For this review, take the finished solid that the model builds, in its own axes (mm). A direction names the side the tool comes from. Coordinates: 2 decimals unless noted, no trailing zeros. Loops run counter-clockwise (first coordinate to the right, second up) from the corner with the lowest first, then second, coordinate; pieces in that order, holes last. Notation, with made-up numbers: (12.25, 56.5) -> (45.25, 56.5) arc R27 ccw to (45.25, 74.5) -> close; hole circle Ø3 at (64, 45). An arc over 180 degrees is marked (long way). One line per item, written item: value.
from build123d import *

# Parameters (mm, degrees)
SKETCH_1_R               = 16.5
EXTRUDE_1_DEPTH          = 2.5
SKETCH_2_R               = 9.5
EXTRUDE_2_DEPTH          = 1.4
SKETCH_3_R               = 1.5
CUT_EXTRUDE_1_DEPTH      = 3
SKETCH_4_R               = 8.5
EXTRUDE_3_DEPTH          = 10
PATTERN_CIRCULAR_1_COUNT = 4
SKETCH_8_R               = 3
EXTRUDE_4_DEPTH          = 6
SKETCH_9_R               = 3.25
CUT_EXTRUDE_2_DEPTH      = 0.5


with BuildPart() as part:
    # 草图1 → 凸台-拉伸1 (new body)
    with BuildSketch(Plane.XY):
        Circle(SKETCH_1_R)
    extrude(amount=EXTRUDE_1_DEPTH)

    # 草图2 → 凸台-拉伸2 (add)
    with BuildSketch(Plane.XY.offset(2.5)):
        Circle(SKETCH_2_R)
    extrude(amount=EXTRUDE_2_DEPTH)

    # 草图3 → 切除-拉伸1 (cut)
    with BuildSketch(Plane.XY.offset(2.5)):
        with Locations((0, 13.5)):
            Circle(SKETCH_3_R)
        with Locations((11.691342951, 6.75)):
            Circle(SKETCH_3_R)
        with Locations((11.691342951, -6.75)):
            Circle(SKETCH_3_R)
        with Locations((0, -13.5)):
            Circle(SKETCH_3_R)
        with Locations((-11.691342951, -6.75)):
            Circle(SKETCH_3_R)
        with Locations((-11.691342951, 6.75)):
            Circle(SKETCH_3_R)
    extrude(amount=-CUT_EXTRUDE_1_DEPTH, mode=Mode.SUBTRACT)

    # 草图4 → 凸台-拉伸3 (add)
    with BuildSketch(Plane.XY.offset(3.9)):
        Circle(SKETCH_4_R)
    extrude(amount=EXTRUDE_3_DEPTH)

    # 草图7 → M3 螺纹孔1 (revolve, cut)
    with BuildSketch(Plane(origin=(0, 6, 13.9), x_dir=(0, -1, 0), z_dir=(1, 0, 0))):
        Polygon((0, 0), (0, 8.401290929), (1.5, 7.5), (1.5, 0), align=None)
    hole_wizard_m3_1 = revolve(axis=Axis((0, 6, 20.25), (0, 0, -1)), mode=Mode.SUBTRACT)

    # 阵列(圆周)1: M3 螺纹孔1 ×4 about axis
    pattern_circular_1_axis = Axis((0, 0, 0), (0, 0, 1))
    for i in range(1, PATTERN_CIRCULAR_1_COUNT):
        add(hole_wizard_m3_1.rotate(pattern_circular_1_axis, i * 360 / PATTERN_CIRCULAR_1_COUNT), mode=Mode.SUBTRACT)

    # 草图8 → 凸台-拉伸4 (add)
    with BuildSketch(Plane.XY.offset(13.9)):
        Circle(SKETCH_8_R)
    extrude(amount=EXTRUDE_4_DEPTH)

    # 草图9 → 切除-拉伸2 (cut)
    with BuildSketch(Plane.XY.offset(2.5)):
        with Locations((0, 13.5)):
            Circle(SKETCH_9_R)
        with Locations((11.691342951, 6.75)):
            Circle(SKETCH_9_R)
        with Locations((11.691342951, -6.75)):
            Circle(SKETCH_9_R)
        with Locations((0, -13.5)):
            Circle(SKETCH_9_R)
        with Locations((-11.691342951, -6.75)):
            Circle(SKETCH_9_R)
        with Locations((-11.691342951, 6.75)):
            Circle(SKETCH_9_R)
    extrude(amount=-CUT_EXTRUDE_2_DEPTH, mode=Mode.SUBTRACT)


solid = part.part
1. Take a section at C-C, the plane z = 12.5. Give the boundary of the cut face in (x, y), and give its area (3 significant figures).
Return value:
outline: circle Ø17 at (0, 0); hole circle Ø3 at (-6, 0); hole circle Ø3 at (0, -6); hole circle Ø3 at (0, 6); hole circle Ø3 at (6, 0)
area: 199 mm2
2. Take a section at D-D, the plane y = -13.5. Give the boundary of the cut face in (x, z), and give its area (3 significant figures).
Return value:
outline: (-9.49, 0) -> (-1.5, 0) -> (-1.5, 2) -> (-3.25, 2) -> (-3.25, 2.5) -> (-9.49, 2.5) -> close; (1.5, 0) -> (9.49, 0) -> (9.49, 2.5) -> (3.25, 2.5) -> (3.25, 2) -> (1.5, 2) -> close
area: 38.2 mm2
3. For faces 4 (the flat face through (12, 5, 2)), 5 (the cylindrical face through (-13.19, 6.82, 1.01)), list the 3-axis set-ups (+Z, -Z, +X, -X, +Y, -Y) from which the entire face can be reached by the end or side of a thin tool; tool diameter is ignored.
Return value:
face 4: +Z
face 5: +Z, -Z
4. Take a section at B-B, the plane x = 12. Give the boundary of the cut face in (y, z).
Return value:
outline: (-11.32, 0) -> (-8.22, 0) -> (-8.22, 2) -> (-9.99, 2) -> (-9.99, 2.5) -> (-11.32, 2.5) -> close; (-5.28, 0) -> (5.28, 0) -> (5.28, 2) -> (3.51, 2) -> (3.51, 2.5) -> (-3.51, 2.5) -> (-3.51, 2) -> (-5.28, 2) -> close; (8.22, 0) -> (11.32, 0) -> (11.32, 2.5) -> (9.99, 2.5) -> (9.99, 2) -> (8.22, 2) -> close
5. The part is to be moulded in two halves that separate along Y. For faces 1 (the cylindrical face through (0, 12, 1)), 2 (the cylindrical face through (15.24, -6.32, 1.23)), 3 (the flat face through (0, 0, 19.9)), say which applies: pulls with the +Y half, pulls with the -Y half, needs draft (parallel to the pull), parting line crosses it, or undercut.
Return value:
face 1: undercut
face 2: parting line crosses it
face 3: needs draft
6. Insertion check: pin 1 Ø5 at (x, y) = (-0.5, 13) entering from +Z; pin 2 Ø10 at (x, y) = (0, 12.5) entering from +Z; pin 3 Ø10 at (y, z) = (-1.5, 10.5) entering from +X; pin 4 Ø2.5 at (x, y) = (-11.69, 6.75) entering from +Z. Each pin has a flat end and moves straight along its axis. Give the tip position at first contact, or say it passes through.
Return value:
pin 1: stops at z = 2
pin 2: stops at z = 13.9
pin 3: stops at x = 8.5
pin 4: passes through
7. Take a section at A-A, the plane z = 1. Give the boundary of the cut face in (x, y).
Return value:
outline: circle Ø33 at (0, 0); hole circle Ø3 at (-11.69, -6.75); hole circle Ø3 at (-11.69, 6.75); hole circle Ø3 at (0, -13.5); hole circle Ø3 at (0, 13.5); hole circle Ø3 at (11.69, -6.75); hole circle Ø3 at (11.69, 6.75)
8. To check wall thickness, follow probe 1 along Y at (x, z) = (0, 0.5); probe 2 along Y at (x, z) = (-1, 10); probe 3 along Z at (x, y) = (-1.5, 7.5). State the ranges of each line that lie inside material, in increasing order. Write a range as from..to.
Return value:
probe 1: y = -16.5..-15, -12..12, 15..16.5
probe 2: y = -8.44..-7.12, -4.88..4.88, 7.12..8.44
probe 3: z = 0..13.9
